from build123d import *

# Parameters (mm, degrees)
F0_W     = 350
F0_H     = 20
F1_DEPTH = 800
F2_W     = 760
F2_H     = 310
F2_W_2   = 720
F2_H_2   = 270
F3_DEPTH = 40
F4_R     = 14.142136
F5_DEPTH = 380


with BuildPart() as f1:
    # F0 (on Right) → F1 (new body)
    with BuildSketch(Plane.YZ):
        with Locations((175, 10)):
            Rectangle(F0_W, F0_H)
    extrude(amount=F1_DEPTH)

    # F2 (on face) → F3 (join)
    with BuildSketch(Plane(origin=(0, 0, 0), x_dir=(1, 0, 0), z_dir=(0, 0, -1))):
        with Locations((400, -175)):
            Rectangle(F2_W, F2_H)
        with Locations((400, -175)):
            Rectangle(F2_W_2, F2_H_2, mode=Mode.SUBTRACT)
    extrude(amount=F3_DEPTH)

    # F4 (on face) → F5 (join)
    with BuildSketch(Plane(origin=(0, 0, 0), x_dir=(1, 0, 0), z_dir=(0, 0, -1))):
        with Locations((30, -30)):
            Circle(F4_R)
        with Locations((770, -30)):
            Circle(F4_R)
        with Locations((30, -320)):
            Circle(F4_R)
        with Locations((770, -320)):
            Circle(F4_R)
    extrude(amount=F5_DEPTH)


solid = f1.part
Could you check a few things on this model? Use its own coordinates, in mm. A direction names the side the tool comes from. Give positions to 0.01 mm unless a question says otherwise; leave off trailing zeros. Order: outer loops, then holes, each group sorted by start corner. A loop starts at its lowest first (then second) coordinate and runs counter-clockwise, first axis right, second up.
Item 1: For faces 5 (the face through (395, 30, -40)), 6 (the face through (777.603, 18.075, -187.34)), 7 (the face through (395, 20, -20)), which set-ups out of +Z, -Z, +X, -X, +Y, -Y let a thin tool reach every point of the face, with its end or its side?
Item 2: If we section it at C-C, the plane y = 30: Write out the boundary of the cut face in (x, z), plus the area to 3 significant figures.
Item 3: I need wall thicknesses on line 1 (X direction, y = 320, z = -218.5); line 2 (Y direction, x = 470, z = -37); line 3 (Z direction, x = 411.5, y = 318). Which ranges of each line are inside material? Lowest first, please.
Item 4: If we section it at A-A, the plane x = 770: Write out the boundary of the cut face in (y, z).
Item 5: If we section it at B-B, the plane z = -276: Write out the boundary of the cut face in (x, y).
Item 6: If we mould it in two halves opening along X, with no side actions, what happens to faces 1 (the face through (20, 177, -20)), 2 (the face through (40, 177, -20)), 3 (the face through (394, 173, 20)), 4 (the face through (780, 177, -20))? For each: pulls with the +X half, pulls with the -X half, needs draft (parallel to the pull), parting line crosses it, or undercut.
Item 7: I'm going to push flat-ended pins straight in: pin 1 (1.5 mm diameter, centred on x = 592.5, y = 49.5, fed in from -Z); pin 2 (22 mm diameter, centred on x = 483.5, y = 320, fed in from -Z); pin 3 (12 mm diameter, centred on y = 215, z = -27, fed in from +X). Where does each tip first touch, or does it pass through?
Values:
1. face 5: -Z, +Y, -Y
1. face 6: -Z
1. face 7: -Z, -Y
2. outline: (0, 0) - (15.86, 0) - (15.86, -380) - (44.14, -380) - (44.14, -40) - (755.86, -40) - (755.86, -380) - (784.14, -380) - (784.14, 0) - (800, 0) - (800, 20) - (0, 20) - close
2. area: 66,000 mm2
3. line 1: x = 15.86 to 44.14, 755.86 to 784.14
3. line 2: y = 20 to 40, 310 to 330
3. line 3: z = -40 to 20
4. outline: (0, 0) - (15.86, 0) - (15.86, -380) - (44.14, -380) - (44.14, -40) - (305.86, -40) - (305.86, -380) - (334.14, -380) - (334.14, 0) - (350, 0) - (350, 20) - (0, 20) - close
5. outline: circle Ø28.28 at (30, 30); circle Ø28.28 at (30, 320); circle Ø28.28 at (770, 30); circle Ø28.28 at (770, 320)
6. face 1: pulls with the -X half
6. face 2: undercut
6. face 3: needs draft
6. face 4: pulls with the +X half
7. pin 1: stops at z = 0
7. pin 2: stops at z = -40
7. pin 3: stops at x = 780
